Verification items for the finished model (mm, model axes). Give positions to 0.01 mm unless a question says otherwise; leave off trailing zeros. Write each loop counter-clockwise with the first axis right and the second up, starting at its lowest first coordinate (ties: lowest second). Pieces come first, ordered by that corner, then holes. Notation, with made-up numbers: (45, 67) - (101, 67) arc R25 ccw to (101, 102) - close; hole circle Ø1 at (39, 89.5). An arc over 180 degrees is marked (long way). Put each result on its own line as item: value.
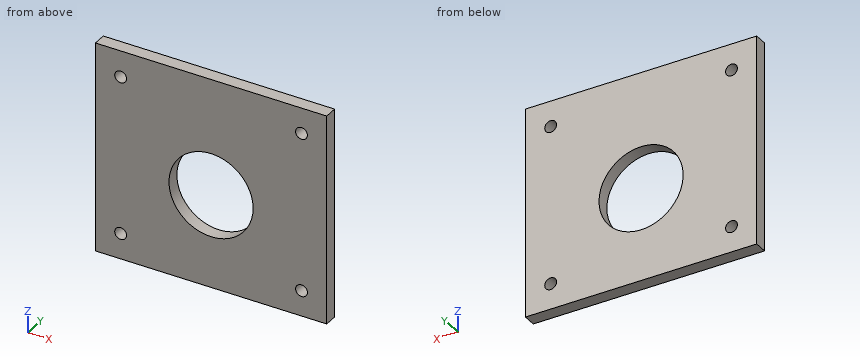
from build123d import *

# Parameters (mm, degrees)
SKETCH_1_W      = 88
SKETCH_1_H      = 80
SKETCH_1_R      = 2.25
SKETCH_1_R_2    = 16
EXTRUDE_1_DEPTH = 5


with BuildPart() as part:
    # Эскиз1 → Бобышка-Вытянуть1 (new body)
    with BuildSketch(Plane(origin=(0, 0, 0), x_dir=(1, 0, 0), z_dir=(0, 1, 0))):
        Rectangle(SKETCH_1_W, SKETCH_1_H)
        with Locations((-34.4, 30.25)):
            Circle(SKETCH_1_R, mode=Mode.SUBTRACT)
        with Locations((34.4, 30.25)):
            Circle(SKETCH_1_R, mode=Mode.SUBTRACT)
        with Locations((34.4, -30.25)):
            Circle(SKETCH_1_R, mode=Mode.SUBTRACT)
        with Locations((-34.4, -30)):
            Circle(SKETCH_1_R, mode=Mode.SUBTRACT)
        with Locations((0, 4.5)):
            Circle(SKETCH_1_R_2, mode=Mode.SUBTRACT)
    extrude(amount=EXTRUDE_1_DEPTH)


solid = part.part
Q1. Section check D-D, the plane x = 34.4. Record the cut outline in (y, z).
Answers follow:
outline: (0, -40) - (5, -40) - (5, -32.5) - (0, -32.5) - close; (0, -28) - (5, -28) - (5, 28) - (0, 28) - close; (0, 32.5) - (5, 32.5) - (5, 40) - (0, 40) - close
Q2. Scan lines: line 1 along Z through (x, y) = (-34.4, 1); line 2 along X through (y, z) = (1.65, 30); line 3 along X through (y, z) = (3.3, 5). Record each from-to range of solid material in increasing order.
Answers follow:
line 1: z = -40 to -32.5, -28 to 27.75, 32.25 to 40
line 2: x = -44 to -36.65, -32.15 to 32.16, 36.64 to 44
line 3: x = -44 to -12.87, 12.87 to 44
Q3. Section check B-B, the plane z = -4.5. Record the cut outline in (x, y).
Answers follow:
outline: (-44, 0) - (-16, 0) - (-16, 5) - (-44, 5) - close; (16, 0) - (44, 0) - (44, 5) - (16, 5) - close
Q4. Section check A-A, the plane x = 0. Record the cut outline in (y, z), plus the area to 3 significant figures.
Answers follow:
outline: (0, -40) - (5, -40) - (5, -20.5) - (0, -20.5) - close; (0, 11.5) - (5, 11.5) - (5, 40) - (0, 40) - close
area: 240 mm2
Q5. Section check C-C, the plane z = -30.25. Record the cut outline in (x, y), plus the area to 3 significant figures.
Answers follow:
outline: (-44, 0) - (-36.65, 0) - (-36.65, 5) - (-44, 5) - close; (-32.15, 0) - (32.15, 0) - (32.15, 5) - (-32.15, 5) - close; (36.65, 0) - (44, 0) - (44, 5) - (36.65, 5) - close
area: 395 mm2
